```python
from build123d import *

# Parameters (mm, degrees)
F0_W      = 66.279934
F0_H      = 140.466083
F1_DEPTH  = 25.4
F2_R      = 13.971168
F3_DEPTH  = 25.4
F4_R      = 19.032879
F5_DEPTH  = 25.4
F5_FACE_R = 19.032879
F6_DEPTH  = 25.4
F7_R      = 18.323501
F7_R_2    = 22.521458
F8_DEPTH  = 25.4


with BuildPart() as f1:
    # F0 (on Front) → F1 (new body)
    with BuildSketch(Plane.XZ):
        with Locations((-19.949931, -13.01357)):
            Rectangle(F0_W, F0_H)
    extrude(amount=F1_DEPTH)

    # F2 (on face) → F3 (cut)
    with BuildSketch(Plane.XZ.offset(25.4)):
        with Locations((-29.521925, 39.461106)):
            Circle(F2_R)
    extrude(amount=-F3_DEPTH, mode=Mode.SUBTRACT)

    # F4 (on face) → F5 (join)
    with BuildSketch(Plane.XZ.offset(25.4)):
        with Locations((-25.564913, -7.869989)):
            Circle(F4_R)
    extrude(amount=F5_DEPTH)

    # F5_face (on face) → F6 (cut)
    with BuildSketch(Plane(origin=(-25.564913, -50.8, -7.869989), x_dir=(1, 0, 0), z_dir=(0, -1, 0))):
        Circle(F5_FACE_R)
    extrude(amount=-F6_DEPTH, mode=Mode.SUBTRACT)

    # F7 (on face) → F8 (cut)
    with BuildSketch(Plane.XZ.offset(25.4)):
        with Locations((-29.70336, -1.401637)):
            Circle(F7_R)
        with Locations((-22.181081, -49.042739)):
            Circle(F7_R_2)
    extrude(amount=-F8_DEPTH, mode=Mode.SUBTRACT)


solid = f1.part
```
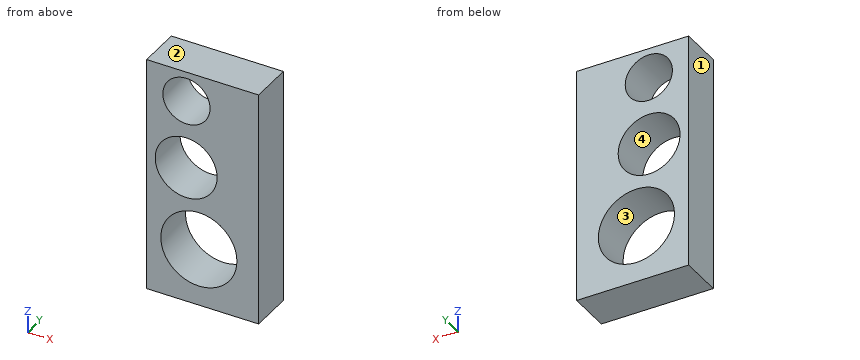
Geometry check sheet. Reference: the model listing, model coordinates, mm. Face numbers are marked on the shaded views. Give positions to 0.01 mm unless a question says otherwise; leave off trailing zeros. Write each loop counter-clockwise with the first axis right and the second up, starting at its lowest first coordinate (ties: lowest second). Pieces come first, ordered by that corner, then holes. Notation, with made-up numbers: (13.5, -31) -> (66.5, -31) arc R31 ccw to (66.5, -6) -> close; hole circle Ø1 at (40.5, 86.25). An arc over 180 degrees is marked (long way). One line per question, with ' | ' between items.
Item 1: Sectioned sample at C-C, the plane x = -13. Record the boundary of the cut face in (y, z).
Determined:
outline: (-25.4, -83.25) -> (0, -83.25) -> (0, -69.61) -> (-25.4, -69.61) -> close; (-25.4, -28.48) -> (0, -28.48) -> (0, -8.93) -> (-25.4, -8.93) -> close; (-25.4, 6.13) -> (0, 6.13) -> (0, 57.22) -> (-25.4, 57.22) -> close
Item 2: Sectioned sample at D-D, the plane y = -6.75. Record the boundary of the cut face in (x, z).
Determined:
outline: (-53.09, -83.25) -> (13.19, -83.25) -> (13.19, 57.22) -> (-53.09, 57.22) -> close; hole circle Ø36.65 at (-29.7, -1.4); hole circle Ø45.04 at (-22.18, -49.04); hole circle Ø27.94 at (-29.52, 39.46)
Item 3: Depth check by flat-ended pin: pin 1 (25 mm diameter, centred on x = -29.52, z = 39.46, fed in from -Y); pin 2 (12 mm diameter, centred on x = -46, z = -1, fed in from +Y). Enter the tip coordinate at first touch or a pass-through.
Determined:
pin 1: through | pin 2: y = 0
Item 4: Scan lines: line 1 along Z through (x, y) = (-42, -15.25); line 2 along Z through (x, y) = (-20, -4.75); line 3 along X through (y, z) = (-18, -51.5). Record each from-to range of solid material in increasing order.
Determined:
line 1: -83.25 to -59.74, -38.35 to -14.99, 12.18 to 33.18, 45.75 to 57.22 | line 2: -83.25 to -71.46, -26.63 to -16.94, 14.14 to 29.24, 49.68 to 57.22 | line 3: -53.09 to -44.57, 0.21 to 13.19
Item 5: Draft check along Z on the marked faces 1, 2, 3 and 4. Enter one of: released by +Z, released by -Z, zero draft, split by the parting line, or undercut.
Determined:
face 1: zero draft | face 2: released by +Z | face 3: undercut | face 4: undercut
Item 6: Sectioned sample at B-B, the plane z = -53. Record the boundary of the cut face in (x, y), plus the area to 3 significant figures.
Determined:
outline: (-53.09, -25.4) -> (-44.35, -25.4) -> (-44.35, 0) -> (-53.09, 0) -> close; (-0.01, -25.4) -> (13.19, -25.4) -> (13.19, 0) -> (-0.01, 0) -> close | area: 557 mm^2
Item 7: Sectioned sample at A-A, the plane x = -26. Record the boundary of the cut face in (y, z), plus the area to 3 significant figures.
Determined:
outline: (-25.4, -83.25) -> (0, -83.25) -> (0, -71.24) -> (-25.4, -71.24) -> close; (-25.4, -26.85) -> (0, -26.85) -> (0, -19.35) -> (-25.4, -19.35) -> close; (-25.4, 16.54) -> (0, 16.54) -> (0, 25.94) -> (-25.4, 25.94) -> close; (-25.4, 52.98) -> (0, 52.98) -> (0, 57.22) -> (-25.4, 57.22) -> close | area: 842 mm^2
